Could you check a few things on this model? Use its own coordinates, in mm. Face numbers are marked on the shaded views. A direction names the side the tool comes from. Give positions to 0.01 mm unless a question says otherwise; leave off trailing zeros. Order: outer loops, then holes, each group sorted by start corner. A loop starts at its lowest first (then second) coordinate and runs counter-clockwise, first axis right, second up. Notation, with made-up numbers: (-18, 61) - (41, 61) arc R28 ccw to (41, 93) - close; hole circle Ø3 at (45.5, 77). An arc over 180 degrees is marked (long way). Put each result on its own line as item: value.
from build123d import *

# Parameters (mm, degrees)
SKETCH_1_W          = 80
SKETCH_1_H          = 60
EXTRUDE_1_DEPTH     = 21.4
FILLET_1_R          = 4.5
CUT_EXTRUDE_1_DEPTH = 77.675595548
SKETCH_3_W          = 76
SKETCH_3_H          = 56
CUT_EXTRUDE_2_DEPTH = 19.4
SKETCH_4_W          = 76
SKETCH_4_H          = 1.3
EXTRUDE_2_DEPTH     = 16.4
CUT_EXTRUDE_3_DEPTH = 26.4
CUT_EXTRUDE_4_REACH = 63.858
SKETCH_6_R          = 1.25
SKETCH_6_R_2        = 1.5
SKETCH_7_R          = 2
CUT_EXTRUDE_5_DEPTH = 1


with BuildPart() as part:
    # 草图1 → 凸台-拉伸1 (new body)
    with BuildSketch(Plane(origin=(0, 0, 0), x_dir=(1, 0, 0), z_dir=(0, 1, 0))):
        with Locations((2.675367047, -10.358890701)):
            Rectangle(SKETCH_1_W, SKETCH_1_H)
    extrude(amount=EXTRUDE_1_DEPTH)

    # 圆角1
    fillet_1_edges = [part.edges().sort_by_distance(p)[0] for p in [
        (2.675367047, 21.4, -19.641109299),
        (2.675367047, 21.4, 40.358890701),
    ]]
    fillet(fillet_1_edges, radius=FILLET_1_R)

    # 草图2 → 切除-拉伸1 (cut, through all)
    with BuildSketch(Plane.XY.offset(40.358890701)):
        Polygon((40.675367047, 21.4), (-35.324632953, 21.4), (-35.324632953, 15.9), (-31.824632953, 11.4), (37.175367047, 11.4), (40.675367047, 15.9), align=None)
    extrude(amount=-CUT_EXTRUDE_1_DEPTH, mode=Mode.SUBTRACT)

    # 草图3 → 切除-拉伸2 (cut)
    with BuildSketch(Plane(origin=(0, 21.4, 0), x_dir=(1, 0, 0), z_dir=(0, 1, 0))):
        with Locations((2.675367047, -10.358890701)):
            Rectangle(SKETCH_3_W, SKETCH_3_H)
    extrude(amount=-CUT_EXTRUDE_2_DEPTH, mode=Mode.SUBTRACT)

    # 草图4 → 凸台-拉伸2 (add)
    with BuildSketch(Plane(origin=(0, 2, 0), x_dir=(1, 0, 0), z_dir=(0, 1, 0))):
        with Locations((2.675367047, -0.808890701)):
            Rectangle(SKETCH_4_W, SKETCH_4_H)
        with Locations((2.675367047, -19.908890701)):
            Rectangle(SKETCH_4_W, SKETCH_4_H)
    extrude(amount=EXTRUDE_2_DEPTH)

    # 草图5 → 切除-拉伸3 (cut)
    with BuildSketch(Plane.XY.offset(20.558890701)):
        Polygon((-32.824984691, 18.4), (-27.324632953, 11.4), (32.675367047, 11.4), (38.175367047, 18.4), align=None)
    extrude(amount=-CUT_EXTRUDE_3_DEPTH, mode=Mode.SUBTRACT)

    # 草图6 → 切除-拉伸4 (cut, up to next)
    with BuildSketch(Plane(origin=(0, 2, 0), x_dir=(1, 0, 0), z_dir=(0, 1, 0)), mode=Mode.PRIVATE) as cut_extrude_4_sk1:
        with Locations(Location((2.675367047, 8.891109299, 0), (0, 0, 270))):
            Circle(SKETCH_6_R)
    cut_extrude_4_tool1 = extrude(cut_extrude_4_sk1.sketch, amount=-CUT_EXTRUDE_4_REACH, mode=Mode.PRIVATE) & part.part
    # 草图6 → 切除-拉伸4 (cut, up to next)
    with BuildSketch(Plane(origin=(0, 2, 0), x_dir=(1, 0, 0), z_dir=(0, 1, 0)), mode=Mode.PRIVATE) as cut_extrude_4_sk2:
        with Locations(Location((2.675367047, -29.608890701, 0), (0, 0, 270))):
            Circle(SKETCH_6_R)
    cut_extrude_4_tool2 = extrude(cut_extrude_4_sk2.sketch, amount=-CUT_EXTRUDE_4_REACH, mode=Mode.PRIVATE) & part.part
    # 草图6 → 切除-拉伸4 (cut, up to next)
    with BuildSketch(Plane(origin=(0, 2, 0), x_dir=(1, 0, 0), z_dir=(0, 1, 0)), mode=Mode.PRIVATE) as cut_extrude_4_sk3:
        with Locations(Location((-25.324632953, 8.891109299, 0), (0, 0, 270))):
            Circle(SKETCH_6_R_2)
    cut_extrude_4_tool3 = extrude(cut_extrude_4_sk3.sketch, amount=-CUT_EXTRUDE_4_REACH, mode=Mode.PRIVATE) & part.part
    # 草图6 → 切除-拉伸4 (cut, up to next)
    with BuildSketch(Plane(origin=(0, 2, 0), x_dir=(1, 0, 0), z_dir=(0, 1, 0)), mode=Mode.PRIVATE) as cut_extrude_4_sk4:
        with Locations(Location((30.675367047, 8.891109299, 0), (0, 0, 270))):
            Circle(SKETCH_6_R_2)
    cut_extrude_4_tool4 = extrude(cut_extrude_4_sk4.sketch, amount=-CUT_EXTRUDE_4_REACH, mode=Mode.PRIVATE) & part.part
    # 草图6 → 切除-拉伸4 (cut, up to next)
    with BuildSketch(Plane(origin=(0, 2, 0), x_dir=(1, 0, 0), z_dir=(0, 1, 0)), mode=Mode.PRIVATE) as cut_extrude_4_sk5:
        with Locations(Location((30.675367047, -10.829122265, 0), (0, 0, 270))):
            Circle(SKETCH_6_R_2)
    cut_extrude_4_tool5 = extrude(cut_extrude_4_sk5.sketch, amount=-CUT_EXTRUDE_4_REACH, mode=Mode.PRIVATE) & part.part
    # 草图6 → 切除-拉伸4 (cut, up to next)
    with BuildSketch(Plane(origin=(0, 2, 0), x_dir=(1, 0, 0), z_dir=(0, 1, 0)), mode=Mode.PRIVATE) as cut_extrude_4_sk6:
        with Locations(Location((30.675367047, -29.608890701, 0), (0, 0, 270))):
            Circle(SKETCH_6_R_2)
    cut_extrude_4_tool6 = extrude(cut_extrude_4_sk6.sketch, amount=-CUT_EXTRUDE_4_REACH, mode=Mode.PRIVATE) & part.part
    # 草图6 → 切除-拉伸4 (cut, up to next)
    with BuildSketch(Plane(origin=(0, 2, 0), x_dir=(1, 0, 0), z_dir=(0, 1, 0)), mode=Mode.PRIVATE) as cut_extrude_4_sk7:
        with Locations(Location((-25.324632953, -29.608890701, 0), (0, 0, 270))):
            Circle(SKETCH_6_R_2)
    cut_extrude_4_tool7 = extrude(cut_extrude_4_sk7.sketch, amount=-CUT_EXTRUDE_4_REACH, mode=Mode.PRIVATE) & part.part
    # 草图6 → 切除-拉伸4 (cut, up to next)
    with BuildSketch(Plane(origin=(0, 2, 0), x_dir=(1, 0, 0), z_dir=(0, 1, 0)), mode=Mode.PRIVATE) as cut_extrude_4_sk8:
        with Locations(Location((-25.324632953, -10.358890701, 0), (0, 0, 270))):
            Circle(SKETCH_6_R_2)
    cut_extrude_4_tool8 = extrude(cut_extrude_4_sk8.sketch, amount=-CUT_EXTRUDE_4_REACH, mode=Mode.PRIVATE) & part.part
    add(cut_extrude_4_tool1.solids().sort_by_distance((2.675367, 2, -8.891109))[0], mode=Mode.SUBTRACT)
    add(cut_extrude_4_tool2.solids().sort_by_distance((2.675367, 2, 29.608891))[0], mode=Mode.SUBTRACT)
    add(cut_extrude_4_tool3.solids().sort_by_distance((-25.324633, 2, -8.891109))[0], mode=Mode.SUBTRACT)
    add(cut_extrude_4_tool4.solids().sort_by_distance((30.675367, 2, -8.891109))[0], mode=Mode.SUBTRACT)
    add(cut_extrude_4_tool5.solids().sort_by_distance((30.675367, 2, 10.829122))[0], mode=Mode.SUBTRACT)
    add(cut_extrude_4_tool6.solids().sort_by_distance((30.675367, 2, 29.608891))[0], mode=Mode.SUBTRACT)
    add(cut_extrude_4_tool7.solids().sort_by_distance((-25.324633, 2, 29.608891))[0], mode=Mode.SUBTRACT)
    add(cut_extrude_4_tool8.solids().sort_by_distance((-25.324633, 2, 10.358891))[0], mode=Mode.SUBTRACT)

    # 草图7 → 切除-拉伸5 (cut)
    with BuildSketch(Plane(origin=(0, 2, 0), x_dir=(1, 0, 0), z_dir=(0, 1, 0))):
        with Locations(Location((-25.324632953, 8.891109299, 0), (0, 0, 270))):
            Circle(SKETCH_7_R)
        with Locations(Location((2.675367047, 8.891109299, 0), (0, 0, 270))):
            Circle(SKETCH_7_R)
        with Locations(Location((30.675367047, 8.891109299, 0), (0, 0, 270))):
            Circle(SKETCH_7_R)
        with Locations(Location((-25.324632953, -10.358890701, 0), (0, 0, 270))):
            Circle(SKETCH_7_R)
        with Locations(Location((30.675367047, -10.829122265, 0), (0, 0, 270))):
            Circle(SKETCH_7_R)
        with Locations(Location((-25.324632953, -29.608890701, 0), (0, 0, 270))):
            Circle(SKETCH_7_R)
        with Locations(Location((2.675367047, -29.608890701, 0), (0, 0, 270))):
            Circle(SKETCH_7_R)
        with Locations(Location((30.675367047, -29.608890701, 0), (0, 0, 270))):
            Circle(SKETCH_7_R)
    extrude(amount=-CUT_EXTRUDE_5_DEPTH, mode=Mode.SUBTRACT)


solid = part.part
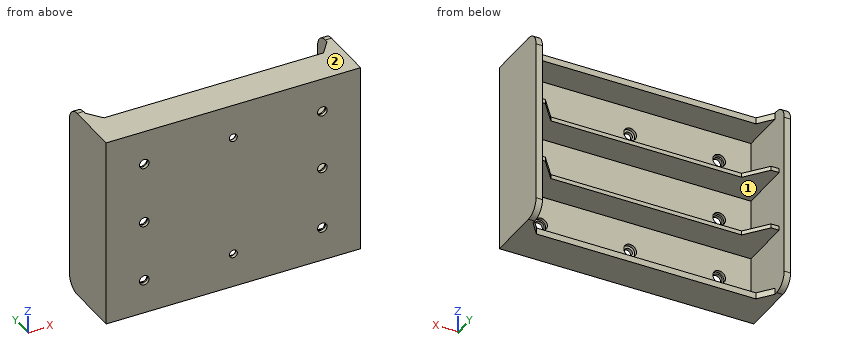
1) Suppose I cut it at D-D, the plane z = -9. State how many separate pieces and enclosed holes the cut face has, and give its area (3 significant figures).
Filled in:
separate pieces: 4
enclosed holes: 0
area: 217 mm^2
2) Suppose I cut it at A-A, the plane x = 14. List the corners of the cut face in (y, z) for me.
Filled in:
outline: (0, -19.64) - (11.4, -19.64) - (11.4, -17.64) - (2, -17.64) - (2, 0.16) - (11.4, 0.16) - (11.4, 1.46) - (2, 1.46) - (2, 19.26) - (11.4, 19.26) - (11.4, 20.56) - (2, 20.56) - (2, 38.36) - (11.4, 38.36) - (11.4, 40.36) - (0, 40.36) - close
3) Suppose I cut it at B-B, the plane z = 25. List the corners of the cut face in (x, y) for me, and give its area (3 significant figures).
Filled in:
outline: (-37.32, 0) - (42.68, 0) - (42.68, 21.4) - (40.68, 21.4) - (40.68, 2) - (-35.32, 2) - (-35.32, 21.4) - (-37.32, 21.4) - close
area: 238 mm^2
4) If I drill on line 1 (Z direction, x = -2.5, y = 3); line 2 (X direction, y = 17.75, z = 31); line 3 (Y direction, x = -10.5, z = 29), over which ranges is the centre line in solid material (lowest first)? Write a range as [from, to].
Filled in:
line 1: z = [-19.64, -17.64], [0.16, 1.46], [19.26, 20.56], [38.36, 40.36]
line 2: x = [-37.32, -35.32], [40.68, 42.68]
line 3: y = [0, 2]
5) I'm going to push flat-ended pins straight in: pin 1 (0.7 mm diameter, centred on x = 14.5, z = 1, fed in from +Y); pin 2 (10 mm diameter, centred on x = 31.5, z = 15, fed in from -Y); pin 3 (1 mm diameter, centred on x = -34, z = 1, fed in from +Y); pin 4 (14 mm diameter, centred on x = 17, z = -8.5, fed in from +Y). Where does each tip first touch, or does it pass through?
Filled in:
pin 1: stops at y = 11.4
pin 2: stops at y = 0
pin 3: stops at y = 18.4
pin 4: stops at y = 2
6) Which directions (+Z, -Z, +X, -X, +Y, -Y) give clear straight access to the entire face, cutting with the end or side of a thin tool? Please do the marked faces 1 and 2.
Filled in:
face 1: +Y
face 2: +Z, +X, -X, +Y, -Y
